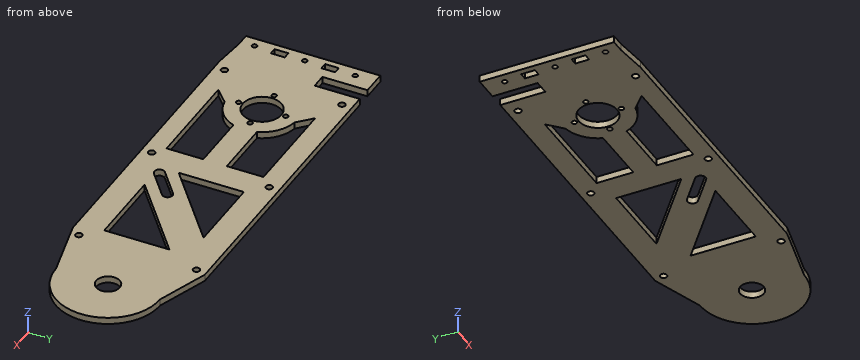
```python
from build123d import *

# Parameters (mm, degrees)
SKETCH_1_R          = 1.5
SKETCH_1_R_2        = 11.5
SKETCH_1_R_3        = 7.04
SKETCH_1_W          = 4.3
SKETCH_1_H          = 8.2
SKETCH_1_H_2        = 8.3
EXTRUDE_1_DEPTH     = 4
SKETCH_2_R          = 2
CUT_EXTRUDE_1_DEPTH = 4


with BuildPart() as part:
    # 草图1 → 凸台-拉伸1 (new body)
    with BuildSketch(Plane.XY):
        with BuildLine():
            Line((-5.457142857, -0.095714286), (-5.457142857, 41.754285714))
            Line((-5.457142857, 41.754285714), (9.542857143, 41.754285714))
            Line((9.542857143, 41.754285714), (9.542857143, 14.904285714))
            Line((9.542857143, 14.904285714), (18.542857143, 14.904285714))
            Line((18.542857143, 14.904285714), (18.542857143, 41.754285714))
            Line((18.542857143, 41.754285714), (199.542857143, 41.754285714))
            Line((199.542857143, 41.754285714), (230.542857143, 30.904285714))
            ThreePointArc((230.542857143, 30.904285714), (261.542857143, -0.095714286), (230.542857143, -31.095714286))
            Line((230.542857143, -31.095714286), (199.556073527, -38.65591431))
            Line((199.556073527, -38.65591431), (192.746868021, -40.245714286))
            Line((192.746868021, -40.245714286), (21.365844759, -40.245714286))
            Line((21.365844759, -40.245714286), (2.692857143, -38.245714286))
            Line((2.692857143, -38.245714286), (-5.457142857, -38.245714286))
            Line((-5.457142857, -38.245714286), (-5.457142857, -0.095714286))
        make_face()
        with Locations((0.542857143, 29.904285714)):
            Circle(SKETCH_1_R, mode=Mode.SUBTRACT)
        with Locations((0.542857143, -0.095714286)):
            Circle(SKETCH_1_R, mode=Mode.SUBTRACT)
        with Locations((0.542857143, -30.095714286)):
            Circle(SKETCH_1_R, mode=Mode.SUBTRACT)
        with Locations((50.542857143, -0.095714286)):
            Circle(SKETCH_1_R_2, mode=Mode.SUBTRACT)
        with Locations((50.542857143, -14.095714286)):
            Circle(SKETCH_1_R, mode=Mode.SUBTRACT)
        with Locations((36.542857143, -0.095714286)):
            Circle(SKETCH_1_R, mode=Mode.SUBTRACT)
        with Locations((50.542857143, 13.904285714)):
            Circle(SKETCH_1_R, mode=Mode.SUBTRACT)
        with Locations((64.542857143, -0.095714286)):
            Circle(SKETCH_1_R, mode=Mode.SUBTRACT)
        with Locations((230.542857143, -0.095714286)):
            Circle(SKETCH_1_R_3, mode=Mode.SUBTRACT)
        with Locations((0.542857143, 14.904285714)):
            Rectangle(SKETCH_1_W, SKETCH_1_H, mode=Mode.SUBTRACT)
        with Locations((0.542857143, -15.145714286)):
            Rectangle(SKETCH_1_W, SKETCH_1_H_2, mode=Mode.SUBTRACT)
    extrude(amount=EXTRUDE_1_DEPTH)

    # 草图2 → 切除-拉伸1 (cut)
    with BuildSketch(Plane.XY.offset(4)):
        with Locations((27.542857143, 35.754285714)):
            Circle(SKETCH_2_R)
        with Locations((112.542857143, 35.754285714)):
            Circle(SKETCH_2_R)
        with Locations((197.542857143, 35.754285714)):
            Circle(SKETCH_2_R)
        with Locations((112.542857143, -34.245714286)):
            Circle(SKETCH_2_R)
        with Locations((197.542857143, -34.245714286)):
            Circle(SKETCH_2_R)
        with Locations((27.542857143, -34.245714286)):
            Circle(SKETCH_2_R)
        Polygon((187.542857143, -24.245714286), (140.41622539, -24.245714286), (187.542857143, 14.56445304), align=None)
        Polygon((122.542857143, 25.754285714), (169.669488896, 25.754285714), (122.542857143, -13.055881612), align=None)
        with BuildLine():
            Line((70.341847016, 6.904285714), (105.542857143, 6.904285714))
            Line((105.542857143, 6.904285714), (105.542857143, 28.754285714))
            Line((105.542857143, 28.754285714), (45.074625519, 28.754285714))
            Line((45.074625519, 28.754285714), (53.568409163, 20.685191252))
            ThreePointArc((53.568409163, 20.685191252), (63.873958655, 16.130244314), (70.341847016, 6.904285714))
        make_face()
        with BuildLine():
            Line((105.542857143, -7.095714286), (105.542857143, -28.945714286))
            Line((105.542857143, -28.945714286), (45.074625519, -28.945714286))
            Line((45.074625519, -28.945714286), (53.568409163, -20.876619824))
            ThreePointArc((53.568409163, -20.876619824), (63.873958655, -16.321672885), (70.341847016, -7.095714286))
            Line((70.341847016, -7.095714286), (105.542857143, -7.095714286))
        make_face()
        with BuildLine():
            Line((125.279005787, -19.870759717), (140.7176105, -7.15661466))
            ThreePointArc((140.7176105, -7.15661466), (144.940522965, -7.565283608), (144.531854017, -11.788196074))
            Line((144.531854017, -11.788196074), (129.093249305, -24.502341131))
            ThreePointArc((129.093249305, -24.502341131), (124.870336839, -24.093672183), (125.279005787, -19.870759717))
        make_face()
    extrude(amount=-CUT_EXTRUDE_1_DEPTH, mode=Mode.SUBTRACT)


solid = part.part
```
Read the model definition and answer for the solid it produces. Units are mm, in the model's axes. Give positions to 0.01 mm unless a question says otherwise; leave off trailing zeros. Loops run counter-clockwise (first coordinate to the right, second up) from the corner with the lowest first, then second, coordinate; pieces in that order, holes last.
Item 1: Each of these flat-tipped pins is pushed along its axis until it touches: pin 1 Ø20.5 at (x, y) = (50.54, -0.1) entering from -Z; pin 2 Ø1.2 at (y, z) = (27, 1) entering from +X. Where does it stop, or does it pass through?
Item 2: The part is cut by section C-C (z = 0.65). Give the number of separate pieces and of enclosed holes in the cut face, and give its area (3 significant figures).
Item 3: Find the intervals of material crossed by line 1 along Y through (x, z) = (144, 1.25); line 2 along Y through (x, z) = (146, 0.25); line 3 along Y through (x, z) = (26, 0.6), in increasing order.
Item 4: The part is cut by section B-B (x = 97.5). Write down the section's boundary in (y, z), and give its area (3 significant figures).
Item 5: The part is cut by section D-D (x = 14.5). Write down the section's boundary in (y, z).
Item 6: The part is cut by section A-A (x = 157). Write down the section's boundary in (y, z).
Taken from the geometry:
1. pin 1: passes through
1. pin 2: stops at x = 246.64
2. separate pieces: 1
2. enclosed holes: 22
2. area: 15,500 mm2
3. line 1: y = -40.25 to -24.25, -21.29 to -12.23, -6.81 to 4.61, 25.75 to 41.75
3. line 2: y = -40.25 to -24.25, -19.65 to 6.26, 25.75 to 41.75
3. line 3: y = -40.25 to -35.52, -32.97 to 34.48, 37.03 to 41.75
4. outline: (-40.25, 0) - (-28.95, 0) - (-28.95, 4) - (-40.25, 4) - close; (-7.1, 0) - (6.9, 0) - (6.9, 4) - (-7.1, 4) - close; (28.75, 0) - (41.75, 0) - (41.75, 4) - (28.75, 4) - close
4. area: 153 mm2
5. outline: (-39.51, 0) - (14.9, 0) - (14.9, 4) - (-39.51, 4) - close
6. outline: (-40.25, 0) - (-24.25, 0) - (-24.25, 4) - (-40.25, 4) - close; (-10.59, 0) - (15.32, 0) - (15.32, 4) - (-10.59, 4) - close; (25.75, 0) - (41.75, 0) - (41.75, 4) - (25.75, 4) - close
